```python
from build123d import *

# Parameters (mm, degrees)
F1_DEPTH = 6.35


with BuildPart() as f1:
    # F0 (on Top) → F1 (new body)
    with BuildSketch(Plane.XY):
        with BuildLine():
            Line((102.076006, 3.715036), (102.076006, 67.215036))
            Line((102.076006, 67.215036), (0.476006, 67.215036))
            ThreePointArc((0.476006, 67.215036), (0.005261, 67.179945), (-0.455078, 67.075446))
            Line((-0.455078, 67.075446), (-97.588172, 37.280782))
            ThreePointArc((-97.588172, 37.280782), (-100.83224, 34.984731), (-102.076006, 31.209964))
            Line((-102.076006, 31.209964), (-102.076006, -57.690036))
            ThreePointArc((-102.076006, -57.690036), (-99.286198, -64.425229), (-92.551006, -67.215036))
            Line((-92.551006, -67.215036), (59.848994, -67.215036))
            ThreePointArc((59.848994, -67.215036), (64.715738, -65.877858), (68.216035, -62.241767))
            Line((68.216035, -62.241767), (100.300694, -3.263398))
            ThreePointArc((100.300694, -3.263398), (101.62522, 0.11468), (102.076006, 3.715036))
        make_face()
    extrude(amount=F1_DEPTH)


solid = f1.part
```
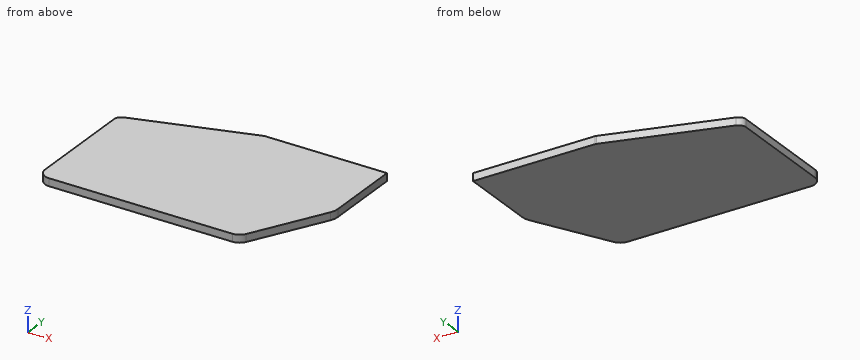
Model file for the job. Use its own axes, mm. Give positions to 0.01 mm unless a question says otherwise; leave off trailing zeros. Loops run counter-clockwise (first coordinate to the right, second up) from the corner with the lowest first, then second, coordinate; pieces in that order, holes last. Notation, with made-up numbers: (0, 83.5) - (11, 83.5) arc R13 ccw to (11, 104.5) - close; hole circle Ø7 at (-24.75, -8). An arc over 180 degrees is marked (long way). One line per item, written item: value. Start each with the question number.
1. Slice it at B-B (y = -16.5). List the corners of the cut face in (x, z).
2. Pin check, flat tips, straight feed: pin 1 (2 mm diameter, centred on x = -26, y = -14.5, fed in from -Z); pin 2 (2 mm diameter, centred on x = -8, z = 5.5, fed in from +Y); pin 3 (3 mm diameter, centred on x = -35, z = 4, fed in from +Y). Stop position of each tip, or through.
3. Slice it at C-C (x = -38.5). List the corners of the cut face in (y, z).
4. Probe L1, parallel to Y at x = 67.5, z = 1.75; L2, parallel to Y at x = -59.5, z = 5.75; L3, parallel to X at y = -20.5, z = 1.25. List the from-to ranges inside material, lowest first. Write a range as from..to.
5. Slice it at A-A (z = 3.5). List the corners of the cut face in (x, y) (3 decimals).
Solution:
1. outline: (-102.08, 0) - (93.1, 0) - (93.1, 6.35) - (-102.08, 6.35) - close
2. pin 1: stops at z = 0
2. pin 2: stops at y = 65.07
2. pin 3: stops at y = 56.94
3. outline: (-67.22, 0) - (55.41, 0) - (55.41, 6.35) - (-67.22, 6.35) - close
4. L1: y = -63.36..67.22
4. L2: y = -67.22..48.96
4. L3: x = -102.08..90.92
5. outline: (-102.076, -57.69) arc R9.525 ccw to (-92.551, -67.215) - (59.849, -67.215) arc R9.525 ccw to (68.216, -62.242) - (100.301, -3.263) arc R14.603 ccw to (102.076, 3.715) - (102.076, 67.215) - (0.476, 67.215) arc R3.175 ccw to (-0.455, 67.075) - (-97.588, 37.281) arc R6.35 ccw to (-102.076, 31.21) - close
